Autodesk Inventor part; units mm, degrees
ref_plane "YZ Plane" through (0, 0, 0) normal (1, 0, 0) x (0, 1, 0)
ref_plane "XZ Plane" through (0, 0, 0) normal (0, 1, 0) x (-1, 0, 0)
ref_plane "XY Plane" through (0, 0, 0) normal (0, 0, 1) x (1, 0, 0)
sketch "Sketch2" plane through (0, 0, 0) normal (1, 0, 0) x (0, 1, 0)
  line L0 (9.7757, 0) -> (-10.7, 0)
  line L1 (27.1787, -1.709) -> (12.4213, -1.709)
  line L2 (10.7, 0) -> (9.7757, 0)
  arc A0 (11, -0.3) -> (10.7, 0) centre (10.7, -0.3) ccw
  line L3 (11, -15) -> (11, -0.3)
  line L4 (-229.8991, 25.4922) -> (33.0555, -2.2844)
  line L5 (72.0462, -3.8892) -> (-254.3637, 30.5904)
  line L6 (33.0555, -2.2844) -> (33.3182, 0.2018)
  line L7 (-27.0281, 6.5763) -> (-27.2907, 4.0901)
  point P0 (0, 0)
  point P1 (33.3182, 0.2018)
  dimension "d5" = 2.5
extrude "Extrusion2" add sketch "Sketch2" along normal mid plane 354.71
ref_plane "Work Plane1" through (-31.6, 28.9, -15.3) normal (0, 0, 1) x (-0.0000001, -1, 0)
sketch "Sketch3" plane through (-100, -27.0281, -15.3) normal (0, 0, 1) x (1, 0, 0)
  circle A0 centre (99.4902, 46.8281) radius 4.4577
  circle A1 centre (122.9497, 46.8285) radius 3.99
  line L0 (144.7507, 45.1805) -> (148.0507, 45.1805)
  circle A2 centre (99.4902, 46.8281) radius 6.5
  circle A3 centre (122.9497, 46.8285) radius 5
  circle A4 centre (146.4007, 46.8285) radius 3.5
  line L1 (148.0507, 48.4805) -> (144.7507, 48.4805)
  line L2 (144.4007, 48.8305) -> (144.4007, 44.8305)
  line L3 (148.0507, 45.1805) -> (148.0507, 48.4805)
  line L4 (144.7507, 45.1805) -> (148.0507, 45.1805)
  line L5 (148.0507, 48.4805) -> (144.7507, 48.4805)
  line L6 (144.7507, 48.4805) -> (144.7507, 45.1805)
  line L7 (149.6507, 50.0785) -> (143.1507, 50.0785)
  line L8 (143.1507, 50.0785) -> (143.1507, 43.5785)
  line L9 (143.1507, 43.5785) -> (149.6507, 43.5785)
  line L10 (149.6507, 43.5785) -> (149.6507, 50.0785)
  line L11 (149.6507, 50.0785) -> (143.1507, 43.5785) construction
  line L12 (143.1507, 50.0785) -> (149.6507, 43.5785) construction
  point P0 (146.4007, 45.1805)
  dimension "d13" = 13
  dimension "d14" = 10
  dimension "d15" = 7
  dimension "d20" = 6.5
  dimension "d21" = 6.5
extrude "Extrusion3" cut sketch "Sketch3" along normal through all contours A0 | A1 | L6 L1 L3 L0 | A2 | A3 | L10 A4 L9 L8 L7 | A4 L7 L10 | L10 L9 A4 | A4 L8 L7 | L9 L8 A4
sketch "Sketch4" plane through (-177.355, -27.2907, 4.0901) normal (0, -0.9944671, 0.1050482) x (1, 0, 0)
  line L0 (354.71, 0) -> (0, 0)
  line L1 (354.71, 2.5) -> (354.71, 0)
  line L2 (0, 2.5) -> (354.71, 2.5)
  line L3 (0, 0) -> (0, 2.5)
  point P0 (177.355, -1.2007)
extrude "Extrusion4" add sketch "Sketch4" along normal blind 600
sketch "Sketch5" plane through (-177.355, 33.3182, 0.2018) normal (0, 0.9944671, -0.1050482) x (1, 0, 0)
  line L0 (0, 0) -> (354.71, 0)
  line L1 (354.71, 2.5) -> (354.71, 0)
  line L2 (0, 2.5) -> (354.71, 2.5)
  line L3 (0, 0) -> (0, 2.5)
  point P0 (177.355, 3.7007)
extrude "Extrusion5" add sketch "Sketch5" along normal blind 72
sketch "Sketch6" plane through (-177.355, -623.7084, 69.6052) normal (0, 0.1050482, 0.9944671) x (1, 0, 0)
  point P0 (177.355, 627.5694)
properties part number "panel"
For this review, take the finished solid that the model builds, in its own axes (mm). Round coordinates to 2 decimals unless told otherwise and drop trailing zeros. Write each loop counter-clockwise with the first axis right and the second up, starting at its lowest first coordinate (ties: lowest second). Pieces come first, ordered by that corner, then holes.
1) Take a section at C-C on z = 38. Give the boundary of the cut face in (x, y) (3 decimals), then the cut area to 3 significant figures.
Answer below:
outline: (-177.355, -348.308) - (177.355, -348.308) - (177.355, -324.509) - (-177.355, -324.509) - close
area: 8,440 mm2
2) Mouldability with a two-part tool opening along Y and no side actions: class faces 1 (the face through (2.49, 25.567, 0.346)), 2 (the face through (177.355, -265, 30)) as +Y half, -Y half, draft (parallel to the pull), parting line (faces both ways), or undercut.
Answer below:
face 1: undercut
face 2: draft
3) Take a section at B-B on y = -87. Give the boundary of the cut face in (x, z) (3 decimals).
Answer below:
outline: (-177.355, 10.397) - (177.355, 10.397) - (177.355, 12.911) - (-177.355, 12.911) - close
4) Take a section at A-A on x = 81.5. Give the boundary of the cut face in (y, z), then the cut area to 3 significant figures.
Answer below:
outline: (-623.97, 67.12) - (104.66, -9.85) - (104.92, -7.36) - (33.32, 0.2) - (-27.03, 6.58) - (-623.71, 69.61) - close
area: 1,830 mm2
5) Insertion check: pin 1 Ø13 at (x, y) = (22.95, 19.8) entering from +Z; pin 2 Ø8 at (y, z) = (-412.5, 37.5) entering from -X; pin 3 Ø17 at (x, y) = (-0.51, 19.8) entering from +Z; pin 4 Ø1 at (x, y) = (2.5, 5.5) entering from -Z. Each pin has a flat end and moves straight along its axis. Give the tip position at first contact, or say it passes through.
Answer below:
pin 1: stops at z = 2.32
pin 2: passes through
pin 3: stops at z = 2.53
pin 4: stops at z = 0.57
6) For line 1 along X through (y, z) = (19.8, 1.45) (3 decimals); line 2 along Z through (x, y) = (79, -303), list the stretches that pass through material, from the lowest coordinate up.
Answer below:
line 1: x = -177.355 to -7.01, 5.99 to 17.95, 27.95 to 43.151, 49.651 to 177.355
line 2: z = 33.21 to 35.73
